Check sheet for the modelled part. Datum: model origin and axes. Units: mm. Give positions to 0.01 mm unless a question says otherwise; leave off trailing zeros. Order: outer loops, then holes, each group sorted by start corner. A loop starts at its lowest first (then second) coordinate and runs counter-clockwise, first axis right, second up. Notation, with made-up numbers: (43, 1.25) -> (73, 1.25) arc R15 ccw to (73, 10.25) -> close; hole circle Ø4 at (12, -24.75). An arc over 180 degrees is marked (long way). Answer in a Markdown table with one row per item. Add a question column.
(1) Cross-section at D-D (x = 95). Record the cut outline in (y, z), then the cut area to 3 significant figures.
(2) Go/stop test with a flat-tipped pin: pin 1 (8 mm diameter, centred on x = 60, y = 60, fed in from -Z). Record where the tip stops, or that it passes through.
(3) Cross-section at A-A (x = 60). Record the cut outline in (y, z), then the cut area to 3 significant figures.
(4) Cross-section at C-C (y = 60). Record the cut outline in (x, z), then the cut area to 3 significant figures.
(5) Cross-section at B-B (z = 11.25). Record the cut outline in (x, y).
(6) Thickness scan on L1, parallel to Y at x = 95, z = 10; L2, parallel to X at y = -2, z = 13.5; L3, parallel to Y at x = 0, z = 4.25. Record the ranges inside material, lowest first. Write a range as [from, to].
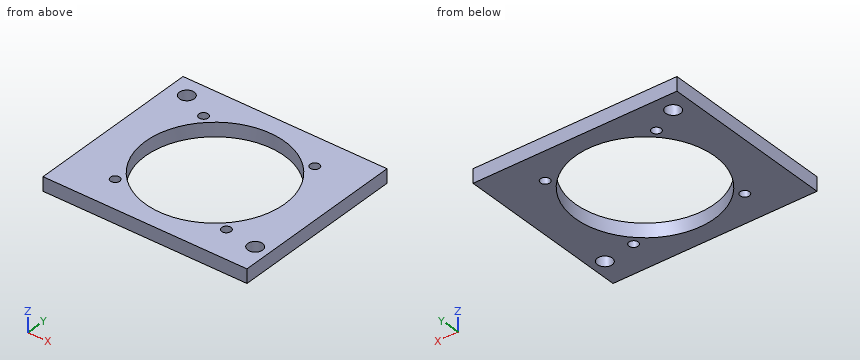
```python
from build123d import *

# Parameters (mm, degrees)
SKETCH1_W           = 220
SKETCH1_H           = 190
BOSS_EXTRUDE1_DEPTH = 15
SKETCH2_R           = 75
SKETCH2_R_2         = 8
SKETCH2_R_3         = 5
CUT_EXTRUDE1_DEPTH  = 15


with BuildPart() as part:
    # Sketch1 → Boss-Extrude1 (new body)
    with BuildSketch(Plane.XY):
        Rectangle(SKETCH1_W, SKETCH1_H)
    extrude(amount=BOSS_EXTRUDE1_DEPTH)

    # Sketch2 → Cut-Extrude1 (cut)
    with BuildSketch(Plane.XY.offset(15)):
        Circle(SKETCH2_R)
        with Locations((-90, 75)):
            Circle(SKETCH2_R_2)
        with Locations(Location((95, -65, 0), (0, 0, 180))):
            Circle(SKETCH2_R_2)
        with Locations((-60, 60)):
            Circle(SKETCH2_R_3)
        with Locations((60, 60)):
            Circle(SKETCH2_R_3)
        with Locations((60, -60)):
            Circle(SKETCH2_R_3)
        with Locations((-60, -60)):
            Circle(SKETCH2_R_3)
    extrude(amount=-CUT_EXTRUDE1_DEPTH, mode=Mode.SUBTRACT)


solid = part.part
```
Answer below:
| question | item | result |
|---|---|---|
| 1 | outline | (-95, 0) -> (-73, 0) -> (-73, 15) -> (-95, 15) -> close; (-57, 0) -> (95, 0) -> (95, 15) -> (-57, 15) -> close |
| 1 | area | 2,610 mm² |
| 2 | pin 1 | passes through |
| 3 | outline | (-95, 0) -> (-65, 0) -> (-65, 15) -> (-95, 15) -> close; (-55, 0) -> (-45, 0) -> (-45, 15) -> (-55, 15) -> close; (45, 0) -> (55, 0) -> (55, 15) -> (45, 15) -> close; (65, 0) -> (95, 0) -> (95, 15) -> (65, 15) -> close |
| 3 | area | 1,200 mm² |
| 4 | outline | (-110, 0) -> (-65, 0) -> (-65, 15) -> (-110, 15) -> close; (-55, 0) -> (-45, 0) -> (-45, 15) -> (-55, 15) -> close; (45, 0) -> (55, 0) -> (55, 15) -> (45, 15) -> close; (65, 0) -> (110, 0) -> (110, 15) -> (65, 15) -> close |
| 4 | area | 1,650 mm² |
| 5 | outline | (-110, -95) -> (110, -95) -> (110, 95) -> (-110, 95) -> close; hole circle Ø16 at (-90, 75); hole circle Ø150 at (0, 0); hole circle Ø10 at (-60, -60); hole circle Ø10 at (-60, 60); hole circle Ø10 at (60, -60); hole circle Ø10 at (60, 60); hole circle Ø16 at (95, -65) |
| 6 | L1 | y = [-95, -73], [-57, 95] |
| 6 | L2 | x = [-110, -74.97], [74.97, 110] |
| 6 | L3 | y = [-95, -75], [75, 95] |
